Verification items for the finished model (mm, model axes). A direction names the side the tool comes from. Give positions to 0.01 mm unless a question says otherwise; leave off trailing zeros. Write each loop counter-clockwise with the first axis right and the second up, starting at its lowest first coordinate (ties: lowest second). Pieces come first, ordered by that corner, then holes. Notation, with made-up numbers: (43.25, 25.5) - (61.25, 25.5) arc R22 cw to (61.25, 45.5) - close; hole circle Ø3 at (36, 34.25). An arc over 180 degrees is marked (long way). Answer as a JSON object with one key per item and string values. Group by question number.
Item 1: Sectioned sample at C-C, the plane x = -7. Record the boundary of the cut face in (y, z), and give its area (4 significant figures).
Item 2: Sectioned sample at B-B, the plane y = 55. Record the boundary of the cut face in (x, z).
Item 3: Draft check along X on faces 1 (the face through (-12.5, 22, -21)), 2 (the face through (3, 31, -7)), 3 (the face through (-13, 60, -14)), 4 (the face through (-4, 2, -3)). Enter one of: +X half, -X half, draft (parallel to the pull), parting line (faces both ways), or undercut.
Item 4: Scan lines: line 1 along X through (y, z) = (6.5, -4); line 2 along Y through (x, z) = (19, -13.5); line 3 along X through (y, z) = (54.5, -29.5). Record each from-to range of solid material in increasing order. Write a range as [from, to].
Item 5: Sectioned sample at A-A, the plane z = -7.5. Record the boundary of the cut face in (x, y), and give its area (3 significant figures).
Item 6: Sectioned sample at D-D, the plane z = -28.5. Record the boundary of the cut face in (x, y), and give its area (3 significant figures).
Item 7: Go/stop test with flat-tipped pins: pin 1 (18.5 mm diameter, centred on y = 14.5, z = -21, fed in from +X); pin 2 (1 mm diameter, centred on x = 20.5, y = -3.5, fed in from -Z); pin 3 (8 mm diameter, centred on x = -8, z = -23.5, fed in from +Y); pin 4 (8 mm diameter, centred on x = 11.5, y = -15.5, fed in from +Z). Record where each tip stops, or that it passes through.
Item 8: Tool access check on faces 5 (the face through (0, 30, -9)), 6 (the face through (21, 3, -7)), 7 (the face through (19, 0, -9)), 8 (the face through (-9, -17.5, -21.2)). Record the directions out of +Z, -Z, +X, -X, +Y, -Y that give a thin tool (end or side, any length) a straight path to the whole face; none if there is none.
```python
from build123d import *

# Parameters (mm, degrees)
F2_DEPTH = 3
F3_DEPTH = 40
F4_DEPTH = 15
F5_SIZE  = 7


with BuildPart() as f2:
    # F1 (on Top) → F2 (new body)
    with BuildSketch(Plane.XY):
        Polygon((0, 60), (-12.5, 60), (-12.5, -21), (38, -21), (38, 0), (0, 0), align=None)
    extrude(amount=-F2_DEPTH)

    # F1 (on Top) → F3 (join)
    with BuildSketch(Plane.XY):
        Polygon((-12.5, -21), (-12.5, 60), (-15.5, 60), (-15.5, -24), (38, -24), (38, -21), align=None)
    extrude(amount=-F3_DEPTH)

    # F1 (on Top) → F4 (join)
    with BuildSketch(Plane.XY):
        Polygon((3, 60), (0, 60), (0, 0), (38, 0), (38, 3), (3, 3), align=None)
    extrude(amount=-F4_DEPTH)

    # F5
    f5_edges = [f2.edges().sort_by_distance(p)[0] for p in [
        (-12.5, -21, -21.5),
    ]]
    chamfer(f5_edges, length=F5_SIZE)


solid = f2.part
```
Geometry check:
{
 "1": {"outline": "(-24, -40) - (-19.5, -40) - (-19.5, -3) - (60, -3) - (60, 0) - (-24, 0) - close", "area": "418.5 mm^2"},
 "2": {"outline": "(-15.5, -40) - (-12.5, -40) - (-12.5, -3) - (0, -3) - (0, -15) - (3, -15) - (3, 0) - (-15.5, 0) - close"},
 "3": {"face 1": "undercut", "face 2": "+X half", "face 3": "draft", "face 4": "undercut"},
 "4": {"line 1": "[-15.5, -12.5], [0, 3]", "line 2": "[-24, -21], [0, 3]", "line 3": "[-15.5, -12.5]"},
 "5": {"outline": "(-15.5, -24) - (38, -24) - (38, -21) - (-5.5, -21) - (-12.5, -14) - (-12.5, 60) - (-15.5, 60) - close; (0, 0) - (38, 0) - (38, 3) - (3, 3) - (3, 60) - (0, 60) - close", "area": "713 mm^2"},
 "6": {"outline": "(-15.5, -24) - (38, -24) - (38, -21) - (-5.5, -21) - (-12.5, -14) - (-12.5, 60) - (-15.5, 60) - close", "area": "428 mm^2"},
 "7": {"pin 1": "x = 3", "pin 2": "z = -3", "pin 3": "y = -14.5", "pin 4": "z = 0"},
 "8": {"face 5": "-Z, +Y", "face 6": "+Z, -Z, +X, +Y", "face 7": "-Z, +X", "face 8": "-Z, +X, +Y"}
}
